Could you check a few things on this model? Use its own coordinates, in mm. A direction names the side the tool comes from. Round coordinates to 2 decimals unless told otherwise and drop trailing zeros. Loops run counter-clockwise (first coordinate to the right, second up) from the corner with the lowest first, then second, coordinate; pieces in that order, holes last. Notation, with made-up numbers: (-2, 60) -> (25, 60) arc R13 cw to (25, 71) -> close; hole circle Ø2 at (-13.75, 47.5). An arc over 180 degrees is marked (long way). One line per item, written item: value.
from build123d import *

# Parameters (mm, degrees)
SKETCH1_R           = 1
BOSS_EXTRUDE1_DEPTH = 0.7
SKETCH2_R           = 1
BOSS_EXTRUDE2_DEPTH = 3.5


with BuildPart() as part:
    # Sketch1 → Boss-Extrude1 (new body)
    with BuildSketch(Plane.XY):
        with BuildLine():
            ThreePointArc((-1.614432161, 2.227214781), (-5.25, 0), (-1.614432161, -2.227214781))
            ThreePointArc((-1.614432161, -2.227214781), (0.086080134, -1.938406924), (1.772413942, -2.300940134))
            ThreePointArc((1.772413942, -2.300940134), (5.25, 0), (1.772413942, 2.300940134))
            ThreePointArc((1.772413942, 2.300940134), (0.086080134, 1.938406924), (-1.614432161, 2.227214781))
        make_face()
        with Locations((-2.75, 0)):
            Circle(SKETCH1_R, mode=Mode.SUBTRACT)
        with Locations((2.75, 0)):
            Circle(SKETCH1_R, mode=Mode.SUBTRACT)
    extrude(amount=BOSS_EXTRUDE1_DEPTH)


with BuildPart() as body_2:
    # Mirror1: mirrored copy
    add(part.part.mirror(Plane(origin=(0, 0, -2.5), x_dir=(1, 0, 0), z_dir=(0, 0, -1))))


with BuildPart() as part_1:
    add(part.part)

    add(body_2.part)  # Boss-Extrude2 merges body 2
    # Sketch2 → Boss-Extrude2 (add, symmetric)
    with BuildSketch(Plane(origin=(0, 0, -2.5), x_dir=(-1, 0, 0), z_dir=(0, 0, -1))):
        with Locations(Location((-2.75, 0, 0), (0, 0, 180))):
            Circle(SKETCH2_R)
        with Locations(Location((2.75, 0, 0), (0, 0, 180))):
            Circle(SKETCH2_R)
    extrude(amount=BOSS_EXTRUDE2_DEPTH, both=True)


solid = part_1.part
(1) If we section it at B-B, the plane x = 4.5: Please give me the cut outline in (y, z), then the cut area to 3 significant figures.
Recorded:
outline: (-1.79, -5.7) -> (1.79, -5.7) -> (1.79, -5) -> (-1.79, -5) -> close; (-1.79, 0) -> (1.79, 0) -> (1.79, 0.7) -> (-1.79, 0.7) -> close
area: 5.00 mm²
(2) If we section it at D-D, the plane z = -4.5: Please give me the cut outline in (x, y).
Recorded:
outline: circle Ø2 at (-2.75, 0); circle Ø2 at (2.75, 0)
(3) If I drill on L1, parallel to Z at x = -1.25, y = -1.75; L2, parallel to Y at x = 0, z = -5.25; L3, parallel to X at y = 0.3, z = -4.25, over which ranges is the centre line in solid material (lowest first)?
Recorded:
L1: -5.7 to -5, 0 to 0.7
L2: -1.94 to 1.94
L3: -3.7 to -1.8, 1.8 to 3.7
(4) For faces 3 (the face through (0, 0, -5)), 4 (the face through (1.96, 0.61, -5.85)), 5 (the face through (0, 0, 0.7)), which set-ups out of +Z, -Z, +X, -X, +Y, -Y let a thin tool reach every point of the face, with its end or its side?
Recorded:
face 3: none
face 4: -Z
face 5: +Z
(5) If we section it at C-C, the plane y = 1.8: Please give me the cut outline in (x, z).
Recorded:
outline: (-4.48, -5.7) -> (4.48, -5.7) -> (4.48, -5) -> (-4.48, -5) -> close; (-4.48, 0) -> (4.48, 0) -> (4.48, 0.7) -> (-4.48, 0.7) -> close
(6) I'm going to push flat-ended pins straight in: pin 1 Ø1.5 at (y, z) = (2, -3) entering from -X; pin 2 Ø1.5 at (x, y) = (-1, 0.5) entering from +Z; pin 3 Ø1.5 at (x, y) = (-0.5, 1) entering from -Z; pin 4 Ø1 at (y, z) = (-1, 0) entering from +X. Where does each tip first touch, or does it pass through?
Recorded:
pin 1: through
pin 2: z = 0.7
pin 3: z = -5.7
pin 4: x = 5.2
(7) Thinking about a two-plate mould opening in X: for faces 1 (the face through (-3.54, 0.61, -5.85)), 2 (the face through (-3, 0, -6)), which applies, released by +X, released by -X, zero draft, split by the parting line, or undercut?
Recorded:
face 1: undercut
face 2: zero draft
